Build history of the part. All positions in model axes, mm. Face numbers are marked on the shaded views. Round coordinates to 2 decimals unless told otherwise and drop trailing zeros. Write each loop counter-clockwise with the first axis right and the second up, starting at its lowest first coordinate (ties: lowest second). Pieces come first, ordered by that corner, then holes. Notation, with made-up numbers: (-24.75, -22.75) -> (-12.75, -22.75) arc R25 cw to (-12.75, -8.75) -> close; hole circle Ø2 at (47, 19). An arc over 180 degrees is marked (long way). Return JSON: item names as keys, results as strings.
from build123d import *

# Parameters (mm, degrees)
CYLINDER001_R     = 1.5
CYLINDER001_DEPTH = 6.8
CYLINDER_R        = 2.5
CYLINDER_DEPTH    = 6.8
BOX002_W          = 34.8
BOX002_H          = 122.8
BOX002_DEPTH      = 1.3
BOX001_W          = 37.4
BOX001_H          = 125.4
BOX001_DEPTH      = 1.3
BOX_W             = 40
BOX_H             = 128
BOX_DEPTH         = 1.3


with BuildPart() as cylinder001:
    # Cylinder001 → Cylinder001 (new body)
    with BuildSketch(Plane(origin=(4.5, 3.8, 0), x_dir=(1, 0, 0), z_dir=(0, 0, 1))):
        Circle(CYLINDER001_R)
    extrude(amount=CYLINDER001_DEPTH)


with BuildPart() as clone003:
    # Clone003 base: copy of Cylinder001
    add(cylinder001.part)


with BuildPart() as clone003_1:
    # Clone003 placement: moved
    add(clone003.part.moved(Location((31, 0, 0))))


with BuildPart() as clone004:
    # Clone004 base: copy of Cylinder001
    add(cylinder001.part)


with BuildPart() as clone004_1:
    # Clone004 placement: moved
    add(clone004.part.moved(Location((0, 113, 0))))


with BuildPart() as board_post_drills:
    # Clone005 base: copy of Cylinder001
    add(cylinder001.part)


with BuildPart() as board_post_drills_1:
    # Clone005 placement: moved
    add(board_post_drills.part.moved(Location((31, 113, 0))))

    # Fusion001: union Cylinder001, Clone003, Clone004
    add(cylinder001.part)
    add(clone003_1.part)
    add(clone004_1.part)


with BuildPart() as cylinder:
    # Cylinder → Cylinder (new body)
    with BuildSketch(Plane(origin=(4.5, 3.8, 0), x_dir=(1, 0, 0), z_dir=(0, 0, 1))):
        Circle(CYLINDER_R)
    extrude(amount=CYLINDER_DEPTH)


with BuildPart() as clone001:
    # Clone001 base: copy of Cylinder
    add(cylinder.part)


with BuildPart() as clone001_1:
    # Clone001 placement: moved
    add(clone001.part.moved(Location((0, 113, 0))))


with BuildPart() as clone:
    # Clone base: copy of Cylinder
    add(cylinder.part)


with BuildPart() as clone_1:
    # Clone placement: moved
    add(clone.part.moved(Location((31, 0, 0))))


with BuildPart() as clone002:
    # Clone002 base: copy of Cylinder
    add(cylinder.part)


with BuildPart() as clone002_1:
    # Clone002 placement: moved
    add(clone002.part.moved(Location((31, 113, 0))))


with BuildPart() as board_posts:
    # Fusion base: copy of Cylinder
    add(cylinder.part)

    # Fusion: union Clone001, Clone, Clone002
    add(clone001_1.part)
    add(clone_1.part)
    add(clone002_1.part)


with BuildPart() as wall_cutout:
    # Box002 → Box002 (new body)
    with BuildSketch(Plane(origin=(2.6, 2.6, 1.3), x_dir=(1, 0, 0), z_dir=(0, 0, 1))):
        with Locations((17.4, 61.4)):
            Rectangle(BOX002_W, BOX002_H)
    extrude(amount=BOX002_DEPTH)


with BuildPart() as wall:
    # Box001 → Box001 (new body)
    with BuildSketch(Plane(origin=(1.3, 1.3, 1.3), x_dir=(1, 0, 0), z_dir=(0, 0, 1))):
        with Locations((18.7, 62.7)):
            Rectangle(BOX001_W, BOX001_H)
    extrude(amount=BOX001_DEPTH)

    # Cut: cut Wall cutout
    add(wall_cutout.part, mode=Mode.SUBTRACT)


with BuildPart() as back_plate_plus_wall_and_posts_drilled:
    # Box → Box (new body)
    with BuildSketch(Plane.XY):
        with Locations((20, 64)):
            Rectangle(BOX_W, BOX_H)
    extrude(amount=BOX_DEPTH)

    # Fusion002: union Board posts, Wall
    add(board_posts.part)
    add(wall.part)

    # Cut001: cut Board post drills
    add(board_post_drills_1.part, mode=Mode.SUBTRACT)


solid = back_plate_plus_wall_and_posts_drilled.part
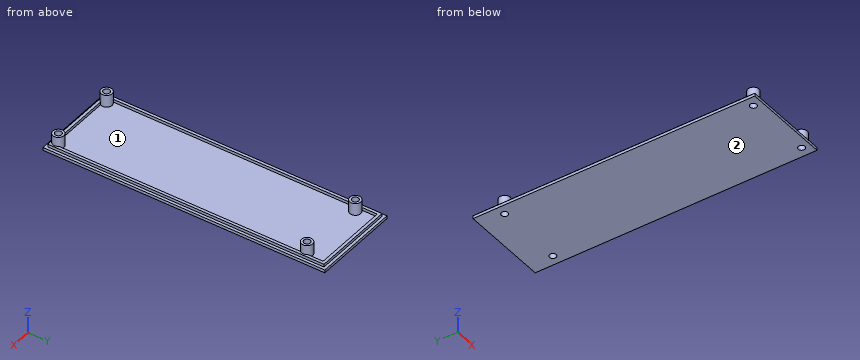
Q1. Two-plate mould, pull along Y, no slides. Class the marked faces 1 and 2: +Y half, -Y half, draft (parallel to the pull), parting line (faces both ways), or undercut.
Verdict:
{"face 1": "undercut", "face 2": "draft"}
Q2. Saw through at B-B on x = 28. List the corners of the cut face in (y, z), then the cut area to 3 significant figures.
Verdict:
{"outline": "(0, 0) -> (128, 0) -> (128, 1.3) -> (126.7, 1.3) -> (126.7, 2.6) -> (125.4, 2.6) -> (125.4, 1.3) -> (2.6, 1.3) -> (2.6, 2.6) -> (1.3, 2.6) -> (1.3, 1.3) -> (0, 1.3) -> close", "area": "170 mm²"}
Q3. Pin check, flat tips, straight feed: pin 1 Ø1 at (x, y) = (4.5, 52) entering from +Z; pin 2 Ø1 at (y, z) = (73, 2) entering from -X; pin 3 Ø1 at (x, z) = (32, 3) entering from +Y. Stop position of each tip, or through.
Verdict:
{"pin 1": "stops at z = 1.3", "pin 2": "stops at x = 1.3", "pin 3": "stops at y = 126.7"}
Q4. Wall check: L1, parallel to Y at x = 35.5, z = 3; L2, parallel to Y at x = 35.5, z = 1.5; L3, parallel to Y at x = 6.5, z = 3.5. Give the ranges that are in metal, low to high.
Verdict:
{"L1": "y = 1.3 to 2.3, 5.3 to 6.3, 114.3 to 115.3, 118.3 to 119.3", "L2": "y = 1.3 to 2.3, 5.3 to 6.3, 114.3 to 115.3, 118.3 to 119.3, 125.4 to 126.7", "L3": "y = 2.3 to 5.3, 115.3 to 118.3"}
Q5. Saw through at C-C on y = 69.5. List the corners of the cut face in (x, z).
Verdict:
{"outline": "(0, 0) -> (40, 0) -> (40, 1.3) -> (38.7, 1.3) -> (38.7, 2.6) -> (37.4, 2.6) -> (37.4, 1.3) -> (2.6, 1.3) -> (2.6, 2.6) -> (1.3, 2.6) -> (1.3, 1.3) -> (0, 1.3) -> close"}
Q6. Saw through at A-A on y = 116.8. List the corners of the cut face in (x, z), then the cut area to 3 significant figures.
Verdict:
{"outline": "(0, 0) -> (3, 0) -> (3, 6.8) -> (2, 6.8) -> (2, 2.6) -> (1.3, 2.6) -> (1.3, 1.3) -> (0, 1.3) -> close; (6, 0) -> (34, 0) -> (34, 6.8) -> (33, 6.8) -> (33, 1.3) -> (7, 1.3) -> (7, 6.8) -> (6, 6.8) -> close; (37, 0) -> (40, 0) -> (40, 1.3) -> (38.7, 1.3) -> (38.7, 2.6) -> (38, 2.6) -> (38, 6.8) -> (37, 6.8) -> close", "area": "68.0 mm²"}
